Input: part model. Units: mm. Frame: model coordinates. Face numbers are marked on the shaded views. A direction names the side the tool comes from. Coordinates: 2 decimals unless noted, no trailing zeros. Write each loop counter-clockwise with the first axis right and the second up, starting at its lowest first coordinate (ties: lowest second). Pieces come first, ordered by that corner, then holes. Notation, with made-up numbers: M 36.5,49 L 86.5,49 A24 ccw 86.5,69 Z; hole C 7.5,76.5 d1. An arc over 180 degrees is marked long. Use CSV: the item, a comma, the result in double quotes.
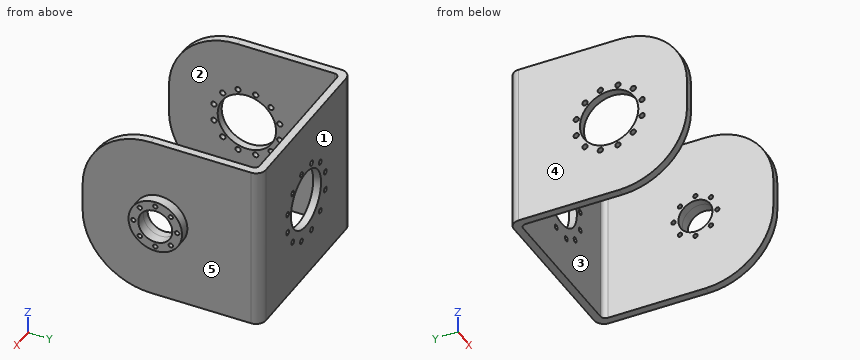
```python
from build123d import *

# Parameters (mm, degrees)
EXTRUDE_1_DEPTH          = 170
SKETCH_2_R               = 30
CUT_EXTRUDE_1_DEPTH      = 180
CUT_EXTRUDE_2_DEPTH      = 304.191358716
CUT_EXTRUDE_2_DEPTH_BACK = 304.191358716
SKETCH_3_R               = 17.5
FILLET_1_R               = 70
FILLET_2_R               = 5
FILLET_3_R               = 10
SKETCH_6_R               = 30
CUT_EXTRUDE_6_DEPTH      = 39
SKETCH_12_R              = 2.75
CUT_EXTRUDE_12_DEPTH     = 10
EXTRUDE_START            = 10.5
SKETCH_14_R              = 27.5
SKETCH_14_R_2            = 17.5
EXTRUDE_2_DEPTH          = 10.5
SKETCH_13_R              = 2.25
CUT_EXTRUDE_13_DEPTH     = 15
SKETCH_15_R              = 2.75
CUT_EXTRUDE_14_DEPTH     = 10


with BuildPart() as part:
    # 草图1 → 凸台-拉伸1 (new body)
    with BuildSketch(Plane.XY):
        Polygon((-164, 0), (0, 0), (0, -175), (8, -175), (8, 8), (-164, 8), (-172, 8), (-172, -175), (-164, -175), align=None)
    extrude(amount=EXTRUDE_1_DEPTH)

    # 草图2 → 切除-拉伸1 (cut)
    with BuildSketch(Plane(origin=(0, 8, 0), x_dir=(1, 0, 0), z_dir=(0, 1, 0))):
        with Locations(Location((-82, -85, 0), (0, 0, 180))):
            Circle(SKETCH_2_R)
    extrude(amount=-CUT_EXTRUDE_1_DEPTH, mode=Mode.SUBTRACT)

    # 草图3 → 切除-拉伸2 (cut, two sides: drawn at the far end of the back side and taken through both)
    with BuildSketch(Plane(origin=(8, 0, 0), x_dir=(0, 0, -1), z_dir=(1, 0, 0)).offset(-CUT_EXTRUDE_2_DEPTH_BACK)):
        with Locations(Location((-85, -95, 0), (0, 0, 90))):
            Circle(SKETCH_3_R)
    extrude(amount=CUT_EXTRUDE_2_DEPTH + CUT_EXTRUDE_2_DEPTH_BACK, mode=Mode.SUBTRACT)

    # 圆角1
    fillet_1_edges = [part.edges().sort_by_distance(p)[0] for p in [
        (4, -175, 0),
        (4, -175, 170),
        (-168, -175, 170),
        (-168, -175, 0),
    ]]
    fillet(fillet_1_edges, radius=FILLET_1_R)

    # 圆角2
    fillet_2_edges = [part.edges().sort_by_distance(p)[0] for p in [
        (0, 0, 85),
        (-164, 0, 85),
    ]]
    fillet(fillet_2_edges, radius=FILLET_2_R)

    # 圆角3
    fillet_3_edges = [part.edges().sort_by_distance(p)[0] for p in [
        (-172, 8, 85),
        (8, 8, 85),
    ]]
    fillet(fillet_3_edges, radius=FILLET_3_R)

    # 草图6 → 切除-拉伸6 (cut)
    with BuildSketch(Plane.ZY.offset(172)):
        with Locations(Location((85, -95, 0), (0, 0, 270))):
            Circle(SKETCH_6_R)
    extrude(amount=-CUT_EXTRUDE_6_DEPTH, mode=Mode.SUBTRACT)

    # 草图12 → 切除-拉伸12 (cut)
    with BuildSketch(Plane.ZY.offset(172)):
        with Locations(Location((94.058666579, -128.80740392, 0), (0, 0, 270))):
            Circle(SKETCH_12_R)
        with Locations(Location((75.941333421, -128.80740392, 0), (0, 0, 270))):
            Circle(SKETCH_12_R)
        with Locations(Location((60.251262658, -119.748737342, 0), (0, 0, 270))):
            Circle(SKETCH_12_R)
        with Locations(Location((51.19259608, -104.058666579, 0), (0, 0, 270))):
            Circle(SKETCH_12_R)
        with Locations(Location((51.19259608, -85.941333421, 0), (0, 0, 270))):
            Circle(SKETCH_12_R)
        with Locations(Location((60.251262658, -70.251262658, 0), (0, 0, 270))):
            Circle(SKETCH_12_R)
        with Locations(Location((75.941333421, -61.19259608, 0), (0, 0, 270))):
            Circle(SKETCH_12_R)
        with Locations(Location((94.058666579, -61.19259608, 0), (0, 0, 270))):
            Circle(SKETCH_12_R)
        with Locations(Location((109.748737342, -70.251262658, 0), (0, 0, 270))):
            Circle(SKETCH_12_R)
        with Locations(Location((118.80740392, -85.941333421, 0), (0, 0, 270))):
            Circle(SKETCH_12_R)
        with Locations(Location((118.80740392, -104.058666579, 0), (0, 0, 270))):
            Circle(SKETCH_12_R)
        with Locations(Location((109.748737342, -119.748737342, 0), (0, 0, 270))):
            Circle(SKETCH_12_R)
    extrude(amount=-CUT_EXTRUDE_12_DEPTH, mode=Mode.SUBTRACT)

    # 草图14 → 凸台-拉伸2 (add)
    with BuildSketch(Plane(origin=(8, 0, 0), x_dir=(0, 0, -1), z_dir=(1, 0, 0)).offset(EXTRUDE_START)):
        with Locations(Location((-85, -95, 0), (0, 0, 270))):
            Circle(SKETCH_14_R)
        with Locations(Location((-85, -95, 0), (0, 0, 90))):
            Circle(SKETCH_14_R_2, mode=Mode.SUBTRACT)
    extrude(amount=-EXTRUDE_2_DEPTH)

    # 草图13 → 切除-拉伸13 (cut, symmetric)
    with BuildSketch(Plane(origin=(8, 0, 0), x_dir=(0, 0, -1), z_dir=(1, 0, 0))):
        with Locations(Location((-85, -72.5, 0), (0, 0, 90))):
            Circle(SKETCH_13_R)
        with Locations(Location((-69.090097423, -79.090097423, 0), (0, 0, 90))):
            Circle(SKETCH_13_R)
        with Locations(Location((-62.5, -95, 0), (0, 0, 90))):
            Circle(SKETCH_13_R)
        with Locations(Location((-69.090097423, -110.909902577, 0), (0, 0, 90))):
            Circle(SKETCH_13_R)
        with Locations(Location((-85, -117.5, 0), (0, 0, 90))):
            Circle(SKETCH_13_R)
        with Locations(Location((-100.909902577, -110.909902577, 0), (0, 0, 90))):
            Circle(SKETCH_13_R)
        with Locations(Location((-107.5, -95, 0), (0, 0, 90))):
            Circle(SKETCH_13_R)
        with Locations(Location((-100.909902577, -79.090097423, 0), (0, 0, 90))):
            Circle(SKETCH_13_R)
    extrude(amount=CUT_EXTRUDE_13_DEPTH, both=True, mode=Mode.SUBTRACT)

    # 草图15 → 切除-拉伸14 (cut)
    with BuildSketch(Plane(origin=(0, 8, 0), x_dir=(1, 0, 0), z_dir=(0, 1, 0))):
        with Locations(Location((-72.941333421, -118.80740392, 0), (0, 0, 270))):
            Circle(SKETCH_15_R)
        with Locations(Location((-93.058666579, -118.80740392, 0), (0, 0, 270))):
            Circle(SKETCH_15_R)
        with Locations(Location((-110.480788149, -108.748737342, 0), (0, 0, 270))):
            Circle(SKETCH_15_R)
        with Locations(Location((-120.539454728, -91.326615771, 0), (0, 0, 270))):
            Circle(SKETCH_15_R)
        with Locations(Location((-120.539454728, -71.209282614, 0), (0, 0, 270))):
            Circle(SKETCH_15_R)
        with Locations(Location((-110.480788149, -53.787161043, 0), (0, 0, 270))):
            Circle(SKETCH_15_R)
        with Locations(Location((-93.058666579, -43.728494465, 0), (0, 0, 270))):
            Circle(SKETCH_15_R)
        with Locations(Location((-72.941333421, -43.728494465, 0), (0, 0, 270))):
            Circle(SKETCH_15_R)
        with Locations(Location((-55.519211851, -53.787161043, 0), (0, 0, 270))):
            Circle(SKETCH_15_R)
        with Locations(Location((-45.460545272, -71.209282614, 0), (0, 0, 270))):
            Circle(SKETCH_15_R)
        with Locations(Location((-45.460545272, -91.326615771, 0), (0, 0, 270))):
            Circle(SKETCH_15_R)
        with Locations(Location((-55.519211851, -108.748737342, 0), (0, 0, 270))):
            Circle(SKETCH_15_R)
    extrude(amount=-CUT_EXTRUDE_14_DEPTH, mode=Mode.SUBTRACT)


solid = part.part
```
1. Access query for the marked faces 1 and 2. Directions: +Z, -Z, +X, -X, +Y, -Y. A direction counts if a zero-diameter tool reaches every point of the face in a straight line with its end or side. Return the directions, or none.
Resolved:
face 1,"+Z, -Z, +X, -X, +Y"
face 2,"+Z, -Z, -Y"
2. Material intervals for line 1 (Y direction, x = 12, z = 85); line 2 (X direction, y = -161.5, z = 112); line 3 (Z direction, x = 3.5, y = -72), sorted ascending. Write a range as [from, to].
Resolved:
line 1,"y = [-122.5, -119.75], [-115.25, -112.5], [-77.5, -74.75], [-70.25, -67.5]"
line 2,"x = [-172, -164], [0, 8]"
line 3,"z = [0, 82.81], [87.19, 170]"
3. Mould query, pull axis X, two halves, no side actions, for the marked faces 3, 4 and 5. Classes: pulls with the +X half, pulls with the -X half, needs draft (parallel to the pull), parting line crosses it, or undercut.
Resolved:
face 3,"undercut"
face 4,"pulls with the -X half"
face 5,"pulls with the +X half"
4. Contact query for flat-ended pins moving along their axis: pin 1 Ø7 at (y, z) = (-61.19, 75.94) entering from +X; pin 2 Ø9 at (x, z) = (-72.94, 43.73) entering from -Y; pin 3 Ø8 at (x, z) = (-1.5, 21) entering from -Y; pin 4 Ø7 at (y, z) = (-95, 62.5) entering from +X. Output: stop coordinate, or through.
Resolved:
pin 1,"stops at x = 8"
pin 2,"stops at y = 0"
pin 3,"stops at y = -158.37"
pin 4,"stops at x = 18.5"
5. Section A-A (y = -12). Return loops of the section in (x, z).
Resolved:
outline,"M -172,0 L -164,0 L -164,170 L -172,170 Z; M 0,0 L 8,0 L 8,170 L 0,170 Z"
6. Section C-C (x = -23). Return loops of the section in (y, z), then the cut area to 3 significant figures.
Resolved:
outline,"M 0,0 L 8,0 L 8,170 L 0,170 Z"
area,"1,360 mm^2"
7. Section D-D (y = -145.5). Return loops of the section in (x, z).
Resolved:
outline,"M -172,12.91 L -164,12.91 L -164,157.09 L -172,157.09 Z; M 0,12.91 L 8,12.91 L 8,157.09 L 0,157.09 Z"
8. Section B-B (z = 30). Return loops of the section in (x, y).
Resolved:
outline,"M -172,-162.45 L -164,-162.45 L -164,-5 A5 cw -159,0 L -5,0 A5 cw 0,-5 L 0,-162.45 L 8,-162.45 L 8,-2 A10 ccw -2,8 L -162,8 A10 ccw -172,-2 Z"
